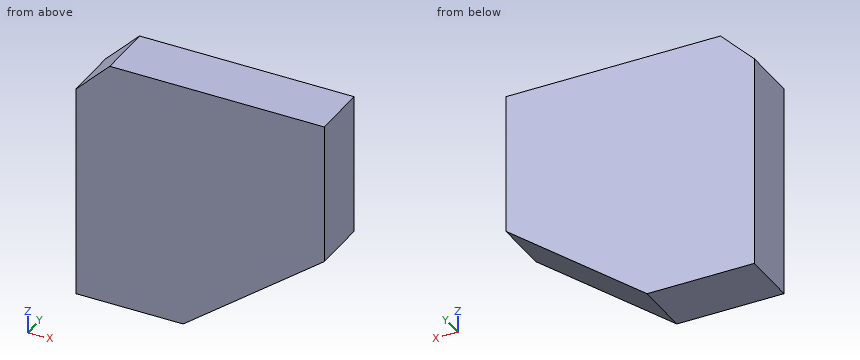
from build123d import *

# Parameters (mm, degrees)
BASE_EXTRUDE_DEPTH = 5
CHAMFER1_SIZE      = 6


with BuildPart() as part:
    # Sketch1 → Base-Extrude (new, symmetric)
    with BuildSketch(Plane(origin=(0, 0, 0), x_dir=(1, 0, 0), z_dir=(0, 1, 0))):
        Polygon((0, 0), (44, 0), (44, 25), (19, 44), (0, 44), align=None)
    extrude(amount=BASE_EXTRUDE_DEPTH, both=True)

    # Chamfer1
    chamfer1_edges = [part.edges().sort_by_distance(p)[0] for p in [
        (0, 0, 0),
    ]]
    chamfer(chamfer1_edges, length=CHAMFER1_SIZE)


solid = part.part
Work out the finished part from the listing and answer in its coordinate system (mm). Give positions to 0.01 mm unless a question says otherwise; leave off trailing zeros. Loops run counter-clockwise (first coordinate to the right, second up) from the corner with the lowest first, then second, coordinate; pieces in that order, holes last. Notation, with made-up numbers: (83, 55) - (101, 55) arc R13 cw to (101, 76) - close; hole circle Ø8 at (33, 35.5). An arc over 180 degrees is marked (long way). Answer in a Markdown table with one row per item.
(1) Section C-C (x = 26) is taken. Give the vertices of the cut face in (y, z).
Results list:
| item | result |
|---|---|
| outline | (-5, -38.68) - (5, -38.68) - (5, 0) - (-5, 0) - close |
(2) Section B-B (x = 37) is taken. Give the vertices of the cut face in (y, z).
Results list:
| item | result |
|---|---|
| outline | (-5, -30.32) - (5, -30.32) - (5, 0) - (-5, 0) - close |
(3) Section A-A (y = -1.25) is taken. Give the vertices of the cut face in (x, z), and give its area (3 significant figures).
Results list:
| item | result |
|---|---|
| outline | (0, -44) - (19, -44) - (44, -25) - (44, 0) - (6, 0) - (0, -6) - close |
| area | 1,680 mm² |
(4) Consider L1, parallel to X at y = 0.25, z = -5.5; L2, parallel to X at y = -2.25, z = -36.5; L3, parallel to Z at x = 27, y = 1.75. Determine where each line is inside the solid, lowest interval first. Write a range as [from, to].
Results list:
| item | result |
|---|---|
| L1 | x = [0.5, 44] |
| L2 | x = [0, 28.87] |
| L3 | z = [-37.92, 0] |
(5) A flat-ended cylindrical pin translates along its axis: pin 1 Ø1 at (x, y) = (26, -0.5) entering from -Z. Find the tip coordinate at first contact, or state that the pin passes through.
Results list:
| item | result |
|---|---|
| pin 1 | stops at z = -39.06 |
